Autodesk Fusion 360 part; units mm, degrees
sketch "Sketch1" plane through (0, 0, 0) normal (1, 0, 0) x (0, 1, 0)
  circle A0 centre (7, 2) radius 2.1
  circle A1 centre (40, 2) radius 2.1
  line L0 (52, -6) -> (0, -6)
  line L1 (52, -6) -> (52, 12)
  circle A2 centre (7, 35) radius 2.6
  line L2 (0, 40) -> (20, 40)
  line L3 (20, 40) -> (20, 25)
  line L4 (20, 25) -> (52, 12)
  line L5 (0, 40) -> (0, -6)
  dimension "d2" = 4.2
  dimension "d4" = 4.2
  dimension "d17" = 52
  dimension "d18" = 5.2
  dimension "d19" = 20
  dimension "d20" = 46
extrude "Extrude1" add sketch "Sketch1" along normal mid plane 8
Check sheet for the modelled part. Datum: model origin and axes. Units: mm. A direction names the side the tool comes from. Give positions to 0.01 mm unless a question says otherwise; leave off trailing zeros. Write each loop counter-clockwise with the first axis right and the second up, starting at its lowest first coordinate (ties: lowest second). Pieces come first, ordered by that corner, then holes. Notation, with made-up numbers: (-30, -34.75) -> (10, -34.75) arc R6 ccw to (10, -24.75) -> close; hole circle Ø1 at (59.5, 45.5). An arc over 180 degrees is marked (long way). Use CSV: the item, a comma, the result in double quotes. Start each with the question number.
Q1. Cross-section at C-C on x = -2. Enter the section's corners in (y, z), and give its area (3 significant figures).
Q2. Depth check by flat-ended pin: P1, Ø2.5, axis at y = 40, z = 2, coming from the +X side; P2, Ø6.5, axis at y = 7, z = 2, coming from the +X side. Enter the tip coordinate at first touch or a pass-through.
Q3. Scan lines: line 1 along Z through (x, y) = (0.5, 7); line 2 along Z through (x, y) = (0, 5.5); line 3 along Y through (x, z) = (-0.5, 33). Record each from-to range of solid material in increasing order.
Q4. Cross-section at D-D on y = 40. Enter the section's corners in (x, z) (3 decimals), and give its area (3 significant figures).
Q5. Cross-section at B-B on z = 2. Enter the section's corners in (x, y), and give its area (3 significant figures).
Q6. Tool access check on faces 1 (the flat face through (-4, 20, 12)), 2 (the flat face through (0, 20, 33)). Record the directions out of +Z, -Z, +X, -X, +Y, -Y that give a thin tool (end or side, any length) a straight path to the whole face; none if there is none.
Q7. Cross-section at A-A on y = 7. Enter the section's corners in (x, z).
Q8. Release check for a two-part mould opening along Y. For faces 3 (the flat face through (-0.06, 35.78, 18.59)), 4 (the cylindrical face through (-0.06, 37.9, 1.91)), 5 (the flat face through (0, 0, 17)) record: +Y half, -Y half, draft (parallel to the pull), parting line (faces both ways), or undercut.
Working result:
1,outline,"(0, -6) -> (52, -6) -> (52, 12) -> (20, 25) -> (20, 40) -> (0, 40) -> close; hole circle Ø5.2 at (7, 35); hole circle Ø4.2 at (7, 2); hole circle Ø4.2 at (40, 2)"
1,area,"1,660 mm^2"
2,P1,"passes through"
2,P2,"stops at x = 4"
3,line 1,"z = -6 to -0.1, 4.1 to 32.4, 37.6 to 40"
3,line 2,"z = -6 to 0.53, 3.47 to 32.88, 37.12 to 40"
3,line 3,"y = 0 to 5.34, 8.66 to 20"
4,outline,"(-4, -6) -> (4, -6) -> (4, -0.1) -> (-4, -0.1) -> close; (-4, 4.1) -> (4, 4.1) -> (4, 16.875) -> (-4, 16.875) -> close"
4,area,"149 mm^2"
5,outline,"(-4, 0) -> (4, 0) -> (4, 4.9) -> (-4, 4.9) -> close; (-4, 9.1) -> (4, 9.1) -> (4, 37.9) -> (-4, 37.9) -> close; (-4, 42.1) -> (4, 42.1) -> (4, 52) -> (-4, 52) -> close"
5,area,"349 mm^2"
6,face 1,"+Z, -Z, -X, +Y, -Y"
6,face 2,"+Z, +X, -X, +Y"
7,outline,"(-4, -6) -> (4, -6) -> (4, -0.1) -> (-4, -0.1) -> close; (-4, 4.1) -> (4, 4.1) -> (4, 32.4) -> (-4, 32.4) -> close; (-4, 37.6) -> (4, 37.6) -> (4, 40) -> (-4, 40) -> close"
8,face 3,"+Y half"
8,face 4,"undercut"
8,face 5,"-Y half"
